```python
from build123d import *

# Parameters (mm, degrees)
SKETCH1_W                = 39
SKETCH1_H                = 7.38
BOSS_EXTRUDE1_DEPTH      = 7.76
SKETCH2_R                = 2.4
CUT_EXTRUDE1_DEPTH       = 7.76
CUT_EXTRUDE2_OUTLINE_R   = 3.1
CUT_EXTRUDE2_OUTLINE_R_2 = 2.4
CUT_EXTRUDE2_DEPTH       = 0.8
CUT_EXTRUDE3_START       = 6.96
CUT_EXTRUDE3_OUTLINE_R   = 3.1
CUT_EXTRUDE3_OUTLINE_R_2 = 2.4
CUT_EXTRUDE3_DEPTH       = 0.8
LPATTERN3_COUNT          = 3
LPATTERN3_PITCH          = 7.79
LPATTERN6_COUNT          = 3
LPATTERN6_PITCH          = 7.79
FILLET1_R                = 3.69
FILLET2_R                = 3.69
FILLET3_R                = 3.69
FILLET4_R                = 3.69
BOSS_EXTRUDE2_START      = -7.76
SKETCH3_R                = 3.1
BOSS_EXTRUDE2_DEPTH      = 7.76
SKETCH4_R                = 3.1
BOSS_EXTRUDE3_DEPTH      = 7.76
SKETCH5_W                = 5.5
SKETCH5_H                = 7.38
BOSS_EXTRUDE5_DEPTH      = 7.76


# Read off the part's stored shape, not the designer's step: Cut-Extrude2, Cut-Extrude3
with BuildPart() as part:
    # Sketch1 → Boss-Extrude1 (new body)
    with BuildSketch(Plane.XY):
        with Locations((19.5, 3.69)):
            Rectangle(SKETCH1_W, SKETCH1_H)
    extrude(amount=BOSS_EXTRUDE1_DEPTH)

    # Sketch2 → Cut-Extrude1 (cut)
    with BuildSketch(Plane.XY.offset(7.76)):
        with Locations((19.5, 3.69)):
            Circle(SKETCH2_R)
    cut_extrude1 = extrude(amount=-CUT_EXTRUDE1_DEPTH, mode=Mode.SUBTRACT)

    # Cut-Extrude2 outline → Cut-Extrude2 (cut)
    with BuildSketch(Plane.XY):
        with Locations((19.5, 3.69)):
            Circle(CUT_EXTRUDE2_OUTLINE_R)
        with Locations((19.5, 3.69)):
            Circle(CUT_EXTRUDE2_OUTLINE_R_2, mode=Mode.SUBTRACT)
    cut_extrude2 = extrude(amount=CUT_EXTRUDE2_DEPTH, mode=Mode.SUBTRACT)

    # Cut-Extrude3 outline → Cut-Extrude3 (cut)
    with BuildSketch(Plane.XY.offset(CUT_EXTRUDE3_START)):
        with Locations((19.5, 3.69)):
            Circle(CUT_EXTRUDE3_OUTLINE_R)
        with Locations((19.5, 3.69)):
            Circle(CUT_EXTRUDE3_OUTLINE_R_2, mode=Mode.SUBTRACT)
    cut_extrude3 = extrude(amount=CUT_EXTRUDE3_DEPTH, mode=Mode.SUBTRACT)

    # LPattern3: Cut-Extrude1, Cut-Extrude2, Cut-Extrude3 ×3
    with Locations(*[(-i * LPATTERN3_PITCH, 0, 0) for i in range(1, LPATTERN3_COUNT)]):
        add(cut_extrude1, mode=Mode.SUBTRACT)
        add(cut_extrude2, mode=Mode.SUBTRACT)
        add(cut_extrude3, mode=Mode.SUBTRACT)

    # LPattern6: Cut-Extrude1, Cut-Extrude2, Cut-Extrude3 ×3
    with Locations(*[(i * LPATTERN6_PITCH, 0, 0) for i in range(1, LPATTERN6_COUNT)]):
        add(cut_extrude1, mode=Mode.SUBTRACT)
        add(cut_extrude2, mode=Mode.SUBTRACT)
        add(cut_extrude3, mode=Mode.SUBTRACT)

    # Fillet1
    fillet1_edges = [part.edges().sort_by_distance(p)[0] for p in [
        (0, 7.38, 3.88),
    ]]
    fillet(fillet1_edges, radius=FILLET1_R)

    # Fillet2
    fillet2_edges = [part.edges().sort_by_distance(p)[0] for p in [
        (0, 0, 3.88),
    ]]
    fillet(fillet2_edges, radius=FILLET2_R - 0.0001)  # a hair under: the kernel refuses the full size

    # Fillet3
    fillet3_edges = [part.edges().sort_by_distance(p)[0] for p in [
        (39, 7.38, 3.88),
    ]]
    fillet(fillet3_edges, radius=FILLET3_R)

    # Fillet4
    fillet4_edges = [part.edges().sort_by_distance(p)[0] for p in [
        (39, 0, 3.88),
    ]]
    fillet(fillet4_edges, radius=FILLET4_R - 0.0001)  # a hair under: the kernel refuses the full size

    # Sketch3 → Boss-Extrude2 (add)
    with BuildSketch(Plane.XY.offset(7.76).offset(BOSS_EXTRUDE2_START)):
        with Locations((3.92, 3.69)):
            Circle(SKETCH3_R)
    extrude(amount=BOSS_EXTRUDE2_DEPTH)

    # Sketch4 → Boss-Extrude3 (add)
    with BuildSketch(Plane(origin=(0, 0, 0), x_dir=(-1, 0, 0), z_dir=(0, 0, -1))):
        with Locations((-35.08, 3.69)):
            Circle(SKETCH4_R)
    extrude(amount=-BOSS_EXTRUDE3_DEPTH)

    # Sketch5 → Boss-Extrude5 (add)
    with BuildSketch(Plane(origin=(0, 0, 0), x_dir=(-1, 0, 0), z_dir=(0, 0, -1))):
        with Locations((-38.06, 3.69)):
            Rectangle(SKETCH5_W, SKETCH5_H)
        with Locations((-0.94, 3.69)):
            Rectangle(SKETCH5_W, SKETCH5_H)
    extrude(amount=-BOSS_EXTRUDE5_DEPTH)


solid = part.part
```
Part model, mm, in its own coordinate system. A direction names the side the tool comes from. Give positions to 0.01 mm unless a question says otherwise; leave off trailing zeros. Write each loop counter-clockwise with the first axis right and the second up, starting at its lowest first coordinate (ties: lowest second). Pieces come first, ordered by that corner, then holes. Notation, with made-up numbers: M 76,-37 L 118,-37 A19 ccw 118,-17 Z; hole C 67,-18 d11. An arc over 180 degrees is marked long. Use CSV: the item, a comma, the result in double quotes.
Item 1: Pull direction X, two halves, no side cores. Call faces 1 (the face through (9, 3, 6.96)), 2 (the face through (40.81, 4, 4)), 3 (the face through (20, 7.38, 4)): +X half, -X half, draft (parallel to the pull), parting line (faces both ways), or undercut.
Taken from the geometry:
face 1,"undercut"
face 2,"+X half"
face 3,"draft"
Item 2: Pin check, flat tip, straight feed: P1, Ø3, axis at x = 27.5, y = 2.5, coming from the -Z side. Stop position of the tip, or through.
Taken from the geometry:
P1,"stops at z = 0.8"
Item 3: Which spindle directions (+Z, -Z, +X, -X, +Y, -Y) get a long thin tool onto all of the face, cutting with end or side? Do faces 4 (the face through (20, 0, 4)), 5 (the face through (20, 1, 6.96)), 6 (the face through (9.25, 1.804, 0.394)). Say none if no direction does.
Taken from the geometry:
face 4,"+Z, -Z, +X, -X, -Y"
face 5,"+Z"
face 6,"-Z"
Item 4: Slice it at C-C on y = 5. State how many separate pieces and enclosed holes the cut face has, plus the area to 3 significant figures.
Taken from the geometry:
separate pieces,"4"
enclosed holes,"0"
area,"229 mm²"
Item 5: Slice it at B-B on z = 3. Write the cut outline in (x, y).
Taken from the geometry:
outline,"M -1.81,0 L 40.81,0 L 40.81,7.38 L -1.81,7.38 Z; hole C 11.71,3.69 d4.8; hole C 19.5,3.69 d4.8; hole C 27.29,3.69 d4.8"
Item 6: Slice it at D-D on x = 11. Write the cut outline in (y, z), plus the area to 3 significant figures.
Taken from the geometry:
outline,"M 0,0 L 0.67,0 L 0.67,0.8 L 1.4,0.8 L 1.4,6.96 L 0.67,6.96 L 0.67,7.76 L 0,7.76 Z; M 5.98,0.8 L 6.71,0.8 L 6.71,0 L 7.38,0 L 7.38,7.76 L 6.71,7.76 L 6.71,6.96 L 5.98,6.96 Z"
area,"19.4 mm²"
Item 7: Drill centre lines: probe 1 along Y at (x, z) = (19.5, 5); probe 2 along X at (y, z) = (4, 4.75); probe 3 along X at (y, z) = (6.25, 7). Where is each one in solid material? Low to high.
Taken from the geometry:
probe 1,"y = 0 to 1.29, 6.09 to 7.38"
probe 2,"x = -1.81 to 9.33, 14.09 to 17.12, 21.88 to 24.91, 29.67 to 40.81"
probe 3,"x = -1.81 to 9.96, 13.46 to 17.75, 21.25 to 25.54, 29.04 to 40.81"
Item 8: Slice it at A-A on x = 27.29. Write the cut outline in (y, z).
Taken from the geometry:
outline,"M 0,0 L 0.59,0 L 0.59,0.8 L 1.29,0.8 L 1.29,6.96 L 0.59,6.96 L 0.59,7.76 L 0,7.76 Z; M 6.09,0.8 L 6.79,0.8 L 6.79,0 L 7.38,0 L 7.38,7.76 L 6.79,7.76 L 6.79,6.96 L 6.09,6.96 Z"
